Here's how the part is built. I have some questions about the finished solid (model axes, mm). A direction names the side the tool comes from. Give positions to 0.01 mm unless a question says otherwise; leave off trailing zeros. Write each loop counter-clockwise with the first axis right and the second up, starting at its lowest first coordinate (ties: lowest second). Pieces come first, ordered by that corner, then holes. Notation, with made-up numbers: (-4, 61) - (16, 61) arc R21 ccw to (16, 73) - close; hole circle Ø1 at (23.25, 85). An arc over 180 degrees is marked (long way). Write each question's results on one line, items separated by ' | '. Start each with the question number.
Item 1: Suppose I cut it at C-C on x = 5. List the corners of the cut face in (y, z) for me (3 decimals), then the cut area to 3 significant figures.
Item 2: Which directions (+Z, -Z, +X, -X, +Y, -Y) give clear straight access to the entire face, cutting with the end or side of a thin tool? Please do faces 5 (the flat face through (3, -247.65, -38)), 6 (the flat face through (3, -103.759, -176)), 7 (the cylindrical face through (1.319, -97.621, -198.605)), 8 (the flat face through (3, -234.95, -16)).
Item 3: Suppose I cut it at D-D on z = -81. List the corners of the cut face in (x, y) for me.
Item 4: Will these pins go through, and if not, where does the flat tip stop? P1, Ø2, axis at x = 4.5, y = -123, coming from the +Z side; P2, Ø3.5, axis at x = 2.5, z = -177, coming from the +Y side; P3, Ø5, axis at y = -63.5, z = -187.325, coming from the +X side; P4, Ø2, axis at x = 5, z = -18.5, coming from the +Y side.
Item 5: Please list where these lines run through material, in increasing order: line 1 along Y through (x, z) = (5.5, -22); line 2 along Y through (x, z) = (2, -176.5); line 3 along Z through (x, y) = (6.25, -236).
Item 6: Suppose I cut it at B-B on z = -196.85. List the corners of the cut face in (x, y) for me, then the cut area to 3 significant figures.
Item 7: Suppose I cut it at A-A on y = -260.35. List the corners of the cut face in (x, z) for me.
Item 8: We'd pull the mould along Y, two halves only. Please class faces 1 (the flat face through (3, -234.95, -99)), 2 (the conical face through (2.85, -98.32, -196.4)), 3 (the flat face through (3, -136.779, -176)), 4 (the flat face through (3, -135, -222.25)): +Y half, -Y half, draft (parallel to the pull), parting line (faces both ways), or undercut.
```python
from build123d import *

# Parameters (mm, degrees)
BOSS_EXTRUDE2_DEPTH                               = 6.604
CSK_FOR_8_FLAT_HEAD_SOCKET_CAP_SCREW1_D           = 4.3053
CSK_FOR_8_FLAT_HEAD_SOCKET_CAP_SCREW1_CSINK_D     = 9.1186
CSK_FOR_8_FLAT_HEAD_SOCKET_CAP_SCREW1_CSINK_ANGLE = 82
CSK_FOR_8_FLAT_HEAD_SOCKET_CAP_SCREW2_D           = 4.3053
CSK_FOR_8_FLAT_HEAD_SOCKET_CAP_SCREW2_CSINK_D     = 9.1186
CSK_FOR_8_FLAT_HEAD_SOCKET_CAP_SCREW2_CSINK_ANGLE = 82
CSK_FOR_1_4_FLAT_HEAD_SOCKET_CAP_SCR_2_COUNT      = 2
CSK_FOR_1_4_FLAT_HEAD_SOCKET_CAP_SCR_2_PITCH      = 214.529804424
CUT_EXTRUDE1_DEPTH                                = 7.604


with BuildPart() as part:
    # Sketch1 → Boss-Extrude2 (new body)
    with BuildSketch(Plane(origin=(0, 0, 0), x_dir=(0, 0, -1), z_dir=(1, 0, 0))):
        with BuildLine():
            Line((0, -234.95), (0, -285.75))
            Line((0, -285.75), (203.2, -285.75))
            ThreePointArc((203.2, -285.75), (216.670384182, -280.170384182), (222.25, -266.7))
            Line((222.25, -266.7), (222.25, 0))
            Line((222.25, 0), (171.45, 0))
            Line((171.45, 0), (171.45, -215.9))
            ThreePointArc((171.45, -215.9), (165.870384182, -229.370384182), (152.4, -234.95))
            Line((152.4, -234.95), (0, -234.95))
        make_face()
    extrude(amount=BOSS_EXTRUDE2_DEPTH)

    # CSK for #8 Flat Head Socket Cap Screw1 (through all)
    with Locations(Plane(origin=(6.604, -103.971373163, -28.9631092), x_dir=(0, 0, 1), z_dir=(1, 0, 0))):
        with Locations((-158.3618908, -91.271373163), (-158.3618908, -40.471373163)):
            CounterSinkHole(CSK_FOR_8_FLAT_HEAD_SOCKET_CAP_SCREW1_D / 2, CSK_FOR_8_FLAT_HEAD_SOCKET_CAP_SCREW1_CSINK_D / 2, counter_sink_angle=CSK_FOR_8_FLAT_HEAD_SOCKET_CAP_SCREW1_CSINK_ANGLE)

    # CSK for #8 Flat Head Socket Cap Screw2 (through all)
    with Locations(Plane(origin=(6.604, 143.822396254, -169.282653802), x_dir=(0, 0, 1), z_dir=(1, 0, 0))):
        with Locations((150.232653802, 391.472396254), (150.232653802, 416.872396254)):
            CounterSinkHole(CSK_FOR_8_FLAT_HEAD_SOCKET_CAP_SCREW2_D / 2, CSK_FOR_8_FLAT_HEAD_SOCKET_CAP_SCREW2_CSINK_D / 2, counter_sink_angle=CSK_FOR_8_FLAT_HEAD_SOCKET_CAP_SCREW2_CSINK_ANGLE)

    # Sketch9 → CSK for 1/4 Flat Head Socket Cap Screw1 (revolve, cut)
    with BuildSketch(Plane(origin=(6.604, -94.869, -196.85), x_dir=(0, 0, -1), z_dir=(0, 1, 0))):
        Polygon((0, 0), (0, 6.604), (3.2639, 6.604), (3.2639, 4.003051983), (6.7437, 0), align=None)
    csk_for_1_4_flat_head_socket_cap_screw1 = revolve(axis=Axis((12.954, -94.869, -196.85), (-1, 0, 0)), mode=Mode.SUBTRACT)

    # CSK for 1_4 Flat Head Socket Cap Scr 2: CSK for 1/4 Flat Head Socket Cap Screw1 ×2
    with Locations(*[Vector(0, -0.771366013, 0.636391761) * (i * CSK_FOR_1_4_FLAT_HEAD_SOCKET_CAP_SCR_2_PITCH) for i in range(1, CSK_FOR_1_4_FLAT_HEAD_SOCKET_CAP_SCR_2_COUNT)]):
        add(csk_for_1_4_flat_head_socket_cap_screw1, mode=Mode.SUBTRACT)

    # Sketch11 → Cut-Extrude1 (cut, through all)
    with BuildSketch(Plane.ZY):
        with BuildLine():
            Line((-171.45, -103.759), (-180.975, -103.759))
            ThreePointArc((-180.975, -103.759), (-183.22006403, -104.68893597), (-184.15, -106.934))
            Line((-184.15, -106.934), (-184.15, -133.604))
            ThreePointArc((-184.15, -133.604), (-183.22006403, -135.84906403), (-180.975, -136.779))
            Line((-180.975, -136.779), (-171.45, -136.779))
            Line((-171.45, -136.779), (-171.45, -103.759))
        make_face()
        with BuildLine():
            Line((-44.45, -234.95), (-31.75, -234.95))
            Line((-31.75, -234.95), (-31.75, -244.475))
            ThreePointArc((-31.75, -244.475), (-32.67993597, -246.72006403), (-34.925, -247.65))
            Line((-34.925, -247.65), (-41.275, -247.65))
            ThreePointArc((-41.275, -247.65), (-43.52006403, -246.72006403), (-44.45, -244.475))
            Line((-44.45, -244.475), (-44.45, -234.95))
        make_face()
    extrude(amount=-CUT_EXTRUDE1_DEPTH, mode=Mode.SUBTRACT)


solid = part.part
```
Checked values:
1) outline: (-285.75, -203.2) arc R19.05 ccw to (-266.7, -222.25) - (0, -222.25) - (0, -171.45) - (-103.759, -171.45) - (-103.759, -180.975) arc R3.175 cw to (-106.934, -184.15) - (-133.604, -184.15) arc R3.175 cw to (-136.779, -180.975) - (-136.779, -171.45) - (-215.9, -171.45) arc R19.05 cw to (-234.95, -152.4) - (-234.95, -44.45) - (-244.475, -44.45) arc R3.175 cw to (-247.65, -41.275) - (-247.65, -34.925) arc R3.175 cw to (-244.475, -31.75) - (-234.95, -31.75) - (-234.95, 0) - (-285.75, 0) - close; hole circle Ø6.33 at (-273.05, -19.05); hole circle Ø10.699 at (-260.35, -60.325); hole circle Ø6.33 at (-247.65, -19.05); hole circle Ø10.699 at (-94.869, -196.85); hole circle Ø6.33 at (-63.5, -187.325); hole circle Ø6.33 at (-12.7, -187.325) | area: 22,300 mm^2
2) face 5: +X, -X, +Y | face 6: +Z, +X, -X | face 7: +X, -X | face 8: +Z, +X, -X, +Y
3) outline: (0, -285.75) - (6.6, -285.75) - (6.6, -234.95) - (0, -234.95) - close
4) P1: stops at z = -184.15 | P2: stops at y = 0 | P3: stops at x = 4.24 | P4: stops at y = -234.95
5) line 1: y = -285.75 to -275.11, -270.99 to -249.71, -245.59 to -234.95 | line 2: y = -285.75 to -136.78, -103.76 to 0 | line 3: z = -222.25 to -44.45, -31.75 to 0
6) outline: (0, -285.75) - (6.6, -285.75) - (6.6, -101.61) - (2.6, -98.13) - (0, -98.13) - close; (0, -91.61) - (2.6, -91.61) - (6.6, -88.13) - (6.6, 0) - (0, 0) - close | area: 1,830 mm^2
7) outline: (0, -222.25) - (6.6, -222.25) - (6.6, -67.07) - (2.6, -63.59) - (0, -63.59) - close; (0, -57.06) - (2.6, -57.06) - (6.6, -53.58) - (6.6, 0) - (0, 0) - close
8) face 1: +Y half | face 2: undercut | face 3: undercut | face 4: draft
